Part model, mm, in its own coordinate system. A direction names the side the tool comes from. Coordinates: 2 decimals unless noted, no trailing zeros. Write each loop counter-clockwise with the first axis right and the second up, starting at its lowest first coordinate (ties: lowest second). Pieces come first, ordered by that corner, then holes. Notation, with made-up numbers: (36, -2) - (40, -2) arc R13 ccw to (40, 15) - close; hole circle Ø2 at (62, 83.5). An arc over 180 degrees is marked (long way). Use a Markdown table: item, result.
```python
from build123d import *

# Parameters (mm, degrees)
BOSS_EXTRUDE1_DEPTH = 25.4
CUT_EXTRUDE1_DEPTH  = 15.875


with BuildPart() as part:
    # Sketch1 → Boss-Extrude1 (new body)
    with BuildSketch(Plane.YZ):
        with BuildLine():
            Line((0, 0), (44.4246, 0))
            Line((44.4246, 0), (44.4246, -19.05))
            Line((44.4246, -19.05), (19.05, -19.05))
            Line((19.05, -19.05), (19.05, -59.6646))
            Line((19.05, -59.6646), (84.9884, -59.6646))
            Line((84.9884, -59.6646), (84.9884, -19.05))
            Line((84.9884, -19.05), (59.6138, -19.05))
            Line((59.6138, -19.05), (59.6138, 0))
            Line((59.6138, 0), (104.0384, 0))
            Line((104.0384, 0), (104.0384, -81.8896))
            Line((104.0384, -81.8896), (58.34888, -81.8896))
            Line((58.34888, -81.8896), (58.34888, -100.9396))
            ThreePointArc((58.34888, -100.9396), (52.013341911, -124.649828033), (45.69968, -100.933765343))
            Line((45.69968, -100.933765343), (45.69968, -81.8896))
            Line((45.69968, -81.8896), (0, -81.8896))
            Line((0, -81.8896), (0, 0))
        make_face()
    extrude(amount=BOSS_EXTRUDE1_DEPTH)

    # Sketch2 → Cut-Extrude1 (cut)
    with BuildSketch(Plane.YZ.offset(25.4)):
        with BuildLine():
            Line((45.69968, -81.8896), (58.34888, -81.8896))
            Line((58.34888, -81.8896), (58.34888, -100.9396))
            ThreePointArc((58.34888, -100.9396), (52.02428, -99.251185541), (45.69968, -100.9396))
            Line((45.69968, -100.9396), (45.69968, -81.8896))
        make_face()
    extrude(amount=-CUT_EXTRUDE1_DEPTH, mode=Mode.SUBTRACT)


solid = part.part
```
Item 1: Drill centre lines: probe 1 along Y at (x, z) = (17, -49.5); probe 2 along Z at (x, y) = (8, 79); probe 3 along Y at (x, z) = (24.25, -5). Where is each one in solid material? Low to high.
From the geometry:
| item | result |
|---|---|
| probe 1 | 0 to 19.05, 84.99 to 104.04 |
| probe 2 | -81.89 to -59.66, -19.05 to 0 |
| probe 3 | 0 to 44.42, 59.61 to 104.04 |
Item 2: Band-saw the part on D-D, the plane x = 3. Give the cut face in (y, z).
From the geometry:
| item | result |
|---|---|
| outline | (0, -81.89) - (45.7, -81.89) - (45.7, -100.93) arc R12.7 ccw (long way) to (58.35, -100.94) - (58.35, -81.89) - (104.04, -81.89) - (104.04, 0) - (59.61, 0) - (59.61, -19.05) - (84.99, -19.05) - (84.99, -59.66) - (19.05, -59.66) - (19.05, -19.05) - (44.42, -19.05) - (44.42, 0) - (0, 0) - close |
Item 3: Drop flat-ended pins along their axis: P1, Ø1, axis at x = 14.5, y = 40, coming from the -Z side; P2, Ø3, axis at x = 6, z = -90.5, coming from the -Y side; P3, Ø3, axis at x = 15, y = 30.5, coming from the -Z side; P4, Ø3, axis at x = 3, y = 88.5, coming from the +Z side. Give the stop position or say it passes through.
From the geometry:
| item | result |
|---|---|
| P1 | z = -117.3 |
| P2 | y = 45.7 |
| P3 | z = -81.89 |
| P4 | z = 0 |
Item 4: Band-saw the part on C-C, the plane z = -16. Give the cut face in (x, y), then the cut area to 3 significant figures.
From the geometry:
| item | result |
|---|---|
| outline | (0, 0) - (25.4, 0) - (25.4, 44.42) - (0, 44.42) - close; (0, 59.61) - (25.4, 59.61) - (25.4, 104.04) - (0, 104.04) - close |
| area | 2,260 mm^2 |
Item 5: Which spindle directions (+Z, -Z, +X, -X, +Y, -Y) get a long thin tool onto all of the face, cutting with end or side? Do faces 1 (the face through (25.4, 53, -68)), 2 (the face through (13, 32, -19.05)), 3 (the face through (13, 59.614, -10)), 4 (the face through (5, 45.7, -92)), 5 (the face through (13, 82, 0)). Say none if no direction does.
From the geometry:
| item | result |
|---|---|
| face 1 | +Z, -Z, +X, +Y, -Y |
| face 2 | +X, -X |
| face 3 | +Z, +X, -X |
| face 4 | +X, -X, -Y |
| face 5 | +Z, +X, -X, +Y, -Y |
Item 6: Two-plate mould, pull along Y, no slides. Class faces 6 (the face through (13, 19.05, -39)), 7 (the face through (5, 58.349, -91)), 8 (the face through (17.57, 52.12, -99.25)), 9 (the face through (13, 53, -81.89)): pulls with the +Y half, pulls with the -Y half, needs draft (parallel to the pull), parting line crosses it, or undercut.
From the geometry:
| item | result |
|---|---|
| face 6 | undercut |
| face 7 | pulls with the +Y half |
| face 8 | parting line crosses it |
| face 9 | needs draft |
Item 7: Band-saw the part on B-B, the plane y = 20.5. Give the cut face in (x, z).
From the geometry:
| item | result |
|---|---|
| outline | (0, -81.89) - (25.4, -81.89) - (25.4, -59.66) - (0, -59.66) - close; (0, -19.05) - (25.4, -19.05) - (25.4, 0) - (0, 0) - close |
